from build123d import *

# Parameters (mm, degrees)
SKETCH1_R           = 101.6
BOSS_EXTRUDE1_DEPTH = 6.35
SKETCH2_R           = 56.642
CUT_EXTRUDE1_DEPTH  = 146.304
SKETCH3_R           = 11.049
CUT_EXTRUDE2_DEPTH  = 146.304
SKETCH4_R           = 11.049
CUT_EXTRUDE3_DEPTH  = 146.304
SKETCH5_R           = 3.175
CUT_EXTRUDE4_DEPTH  = 146.304
BOSS_EXTRUDE2_START = 6.35
SKETCH6_R           = 101.6
SKETCH6_R_2         = 97.155
BOSS_EXTRUDE2_DEPTH = 6.35


with BuildPart() as part:
    # Sketch1 → Boss-Extrude1 (new body)
    with BuildSketch(Plane.XY):
        Circle(SKETCH1_R)
    extrude(amount=BOSS_EXTRUDE1_DEPTH)

    # Sketch2 → Cut-Extrude1 (cut)
    with BuildSketch(Plane.XY.offset(6.35)):
        Circle(SKETCH2_R)
    extrude(amount=-CUT_EXTRUDE1_DEPTH, mode=Mode.SUBTRACT)

    # Sketch3 → Cut-Extrude2 (cut)
    with BuildSketch(Plane.XY.offset(6.35)):
        with Locations((0, 72.644)):
            Circle(SKETCH3_R)
        with Locations((42.699071868, 58.770230539)):
            Circle(SKETCH3_R)
        with Locations((69.08854957, 22.448230539)):
            Circle(SKETCH3_R)
        with Locations((69.08854957, -22.448230539)):
            Circle(SKETCH3_R)
        with Locations((42.699071868, -58.770230539)):
            Circle(SKETCH3_R)
        with Locations((0, -72.644)):
            Circle(SKETCH3_R)
        with Locations((-42.699071868, -58.770230539)):
            Circle(SKETCH3_R)
        with Locations((-69.08854957, -22.448230539)):
            Circle(SKETCH3_R)
        with Locations((-69.08854957, 22.448230539)):
            Circle(SKETCH3_R)
        with Locations((-42.699071868, 58.770230539)):
            Circle(SKETCH3_R)
    extrude(amount=-CUT_EXTRUDE2_DEPTH, mode=Mode.SUBTRACT)

    # Sketch4 → Cut-Extrude3 (cut)
    with BuildSketch(Plane.XY.offset(6.35)):
        with Locations((84.074, 0)):
            Circle(SKETCH4_R)
        with Locations((68.017294785, -49.417457301)):
            Circle(SKETCH4_R)
        with Locations((25.980294785, -79.959125551)):
            Circle(SKETCH4_R)
        with Locations((-25.980294785, -79.959125551)):
            Circle(SKETCH4_R)
        with Locations((-68.017294785, -49.417457301)):
            Circle(SKETCH4_R)
        with Locations((-84.074, 0)):
            Circle(SKETCH4_R)
        with Locations((-68.017294785, 49.417457301)):
            Circle(SKETCH4_R)
        with Locations((-25.980294785, 79.959125551)):
            Circle(SKETCH4_R)
        with Locations((25.980294785, 79.959125551)):
            Circle(SKETCH4_R)
        with Locations((68.017294785, 49.417457301)):
            Circle(SKETCH4_R)
    extrude(amount=-CUT_EXTRUDE3_DEPTH, mode=Mode.SUBTRACT)

    # Sketch5 → Cut-Extrude4 (cut)
    with BuildSketch(Plane.XY.offset(6.35)):
        with Locations((53.867555897, 40.259)):
            Circle(SKETCH5_R)
        with Locations((-53.828444103, 40.259)):
            Circle(SKETCH5_R)
        with Locations((-53.828444103, -40.259)):
            Circle(SKETCH5_R)
        with Locations((53.867555897, -40.259)):
            Circle(SKETCH5_R)
    extrude(amount=-CUT_EXTRUDE4_DEPTH, mode=Mode.SUBTRACT)

    # Sketch6 → Boss-Extrude2 (add)
    with BuildSketch(Plane(origin=(0, 0, 0), x_dir=(-1, 0, 0), z_dir=(0, 0, -1)).offset(BOSS_EXTRUDE2_START)):
        Circle(SKETCH6_R)
        Circle(SKETCH6_R_2, mode=Mode.SUBTRACT)
    extrude(amount=-BOSS_EXTRUDE2_DEPTH)


solid = part.part
Check sheet for the modelled part. Datum: model origin and axes. Units: mm. A direction names the side the tool comes from. Give positions to 0.01 mm unless a question says otherwise; leave off trailing zeros. Write each loop counter-clockwise with the first axis right and the second up, starting at its lowest first coordinate (ties: lowest second). Pieces come first, ordered by that corner, then holes. Notation, with made-up numbers: (73, 34.5) -> (131, 34.5) arc R10 ccw to (131, 43.5) -> close; hole circle Ø5 at (3, 41). An arc over 180 degrees is marked (long way). One line per item, written item: value. Start each with the question number.
Item 1: Tool access check on faces 1 (the flat face through (-36, 44, 0)), 2 (the cylindrical face through (-15.44, -76.64, 3.22)). Record the directions out of +Z, -Z, +X, -X, +Y, -Y that give a thin tool (end or side, any length) a straight path to the whole face; none if there is none.
Item 2: Gauge pin test, flat ends, axial feed: pin 1 (5 mm diameter, centred on x = 45, z = 2.5, fed in from +Y); pin 2 (5 mm diameter, centred on x = -53.83, y = 40.26, fed in from +Z); pin 3 (1.5 mm diameter, centred on y = 79, z = 2, fed in from +X); pin 4 (1.5 mm diameter, centred on y = -74.5, z = 2, fed in from +X). Record the tip position at first contact, or that the pin passes through.
Item 3: Section check D-D on z = -2. Record the cut outline in (x, y) (3 decimals).
Item 4: Material ranges on probe 1 along X at (y, z) = (-15, 5.25); probe 2 along X at (y, z) = (-2.5, 5.5); probe 3 along Y at (x, z) = (-33.5, 2.25), recorded low to high. Write a range as from..to.
Item 5: Section check A-A on x = 0. Record the cut outline in (y, z) (3 decimals).
Item 6: Section check C-C on x = 60.5. Record the cut outline in (y, z), then the cut area to 3 significant figures.
Item 7: Section check B-B on y = 0. Record the cut outline in (x, z) (3 decimals).
Item 8: Draft check along X on faces 3 (the flat face through (-82.3, -52.2, -6.35)), 4 (the cylindrical face through (47.8, -68.57, 3.22)). Enter one of: +X half, -X half, draft (parallel to the pull), parting line (faces both ways), or undercut.
Results list:
1. face 1: -Z
1. face 2: +Z, -Z
2. pin 1: y = 92.28
2. pin 2: through
2. pin 3: x = 64.8
2. pin 4: x = 69.88
3. outline: circle Ø203.2 at (0, 0); hole circle Ø194.31 at (0, 0)
4. probe 1: -100.49..-77.25, -60.93..-54.62, 54.62..60.93, 77.25..100.49
4. probe 2: -101.57..-94.84, -73.31..-56.59, 56.59..73.31, 94.84..101.57
4. probe 3: -95.92..-88.05, -71.86..-64.89, -52.65..-45.67, 45.67..52.65, 64.89..71.86, 88.05..95.92
5. outline: (-101.6, -6.35) -> (-97.155, -6.35) -> (-97.155, 0) -> (-83.693, 0) -> (-83.693, 6.35) -> (-101.6, 6.35) -> close; (-61.595, 0) -> (-56.642, 0) -> (-56.642, 6.35) -> (-61.595, 6.35) -> close; (56.642, 0) -> (61.595, 0) -> (61.595, 6.35) -> (56.642, 6.35) -> close; (83.693, 0) -> (97.155, 0) -> (97.155, -6.35) -> (101.6, -6.35) -> (101.6, 6.35) -> (83.693, 6.35) -> close
6. outline: (-81.62, -6.35) -> (-76.02, -6.35) -> (-76.02, 0) -> (-57.52, 0) -> (-57.52, 6.35) -> (-81.62, 6.35) -> close; (-41.32, 0) -> (-29.4, 0) -> (-29.4, 6.35) -> (-41.32, 6.35) -> close; (-15.5, 0) -> (15.5, 0) -> (15.5, 6.35) -> (-15.5, 6.35) -> close; (29.4, 0) -> (41.32, 0) -> (41.32, 6.35) -> (29.4, 6.35) -> close; (57.52, 0) -> (76.02, 0) -> (76.02, -6.35) -> (81.62, -6.35) -> (81.62, 6.35) -> (57.52, 6.35) -> close
6. area: 726 mm²
7. outline: (-101.6, -6.35) -> (-97.155, -6.35) -> (-97.155, 0) -> (-95.123, 0) -> (-95.123, 6.35) -> (-101.6, 6.35) -> close; (-73.025, 0) -> (-56.642, 0) -> (-56.642, 6.35) -> (-73.025, 6.35) -> close; (56.642, 0) -> (73.025, 0) -> (73.025, 6.35) -> (56.642, 6.35) -> close; (95.123, 0) -> (97.155, 0) -> (97.155, -6.35) -> (101.6, -6.35) -> (101.6, 6.35) -> (95.123, 6.35) -> close
8. face 3: draft
8. face 4: undercut
